from build123d import *

# Parameters (mm, degrees)
SKETCH1_W               = 32
SKETCH1_H               = 80
BOSS_EXTRUDE1_DEPTH     = 3
SKETCH4_W               = 32
SKETCH4_H               = 80
SKETCH4_W_2             = 27
SKETCH4_H_2             = 74
BOSS_EXTRUDE2_DEPTH     = 57.5
SKETCH5_W               = 32
SKETCH5_H               = 140
BOSS_EXTRUDE3_DEPTH     = 2.5
CUT_EXTRUDE1_DEPTH      = 50.8
CUT_EXTRUDE1_DEPTH_BACK = 94.573500522
SKETCH2_W               = 22
SKETCH2_H               = 41
SKETCH6_R               = 3.25
SKETCH6_W               = 22
SKETCH6_H               = 74
CUT_EXTRUDE2_DEPTH      = 25.4
CUT_EXTRUDE3_DEPTH      = 100.463561167
CUT_EXTRUDE3_DEPTH_BACK = 100.463561167
SKETCH8_W               = 74
SKETCH8_H               = 60
SKETCH7_R               = 2
CUT_EXTRUDE4_DEPTH      = 94.573500522
SKETCH10_W              = 2
SKETCH10_H              = 140
CUT_EXTRUDE5_DEPTH      = 96.524865873
FILLET1_R               = 5
SKETCH13_W              = 3
SKETCH13_H              = 41
CUT_EXTRUDE7_DEPTH      = 94.252345815


with BuildPart() as part:
    # Sketch1 → Boss-Extrude1 (new body)
    with BuildSketch(Plane(origin=(0, 0, 0), x_dir=(1, 0, 0), z_dir=(0, 1, 0))):
        with Locations((0, 9)):
            Rectangle(SKETCH1_W, SKETCH1_H)
    extrude(amount=BOSS_EXTRUDE1_DEPTH)

    # Sketch4 → Boss-Extrude2 (add)
    with BuildSketch(Plane(origin=(0, 3, 0), x_dir=(1, 0, 0), z_dir=(0, 1, 0))):
        with Locations((0, 9)):
            Rectangle(SKETCH4_W, SKETCH4_H)
        with Locations((0, 9)):
            Rectangle(SKETCH4_W_2, SKETCH4_H_2, mode=Mode.SUBTRACT)
    extrude(amount=BOSS_EXTRUDE2_DEPTH)

    # Sketch5 → Boss-Extrude3 (add)
    with BuildSketch(Plane(origin=(0, 60.5, 0), x_dir=(1, 0, 0), z_dir=(0, 1, 0))):
        Rectangle(SKETCH5_W, SKETCH5_H)
    extrude(amount=BOSS_EXTRUDE3_DEPTH)

    # Sketch2 → Cut-Extrude1 (cut, two sides: drawn at the far end of the back side and taken through both)
    with BuildSketch(Plane(origin=(0, 3, 0), x_dir=(1, 0, 0), z_dir=(0, 1, 0)).offset(-CUT_EXTRUDE1_DEPTH_BACK)):
        with Locations((0, 9)):
            Rectangle(SKETCH2_W, SKETCH2_H)
    extrude(amount=CUT_EXTRUDE1_DEPTH + CUT_EXTRUDE1_DEPTH_BACK, mode=Mode.SUBTRACT)

    # Sketch6 → Cut-Extrude2 (cut)
    with BuildSketch(Plane(origin=(0, 63, 0), x_dir=(1, 0, 0), z_dir=(0, 1, 0))):
        with Locations(Location((0, 63.5, 0), (0, 0, 270))):
            Circle(SKETCH6_R)
        with Locations(Location((0, -63.5, 0), (0, 0, 270))):
            Circle(SKETCH6_R)
        with Locations((0, 9)):
            Rectangle(SKETCH6_W, SKETCH6_H)
    extrude(amount=-CUT_EXTRUDE2_DEPTH, mode=Mode.SUBTRACT)

    # Sketch8 → Cut-Extrude3 (cut, two sides: drawn at the far end of the back side and taken through both)
    with BuildSketch(Plane(origin=(16, 0, 0), x_dir=(0, 0, -1), z_dir=(1, 0, 0)).offset(-CUT_EXTRUDE3_DEPTH_BACK)):
        with Locations((9, 33)):
            Rectangle(SKETCH8_W, SKETCH8_H)
    extrude(amount=CUT_EXTRUDE3_DEPTH + CUT_EXTRUDE3_DEPTH_BACK, mode=Mode.SUBTRACT)

    # Sketch7 → Cut-Extrude4 (cut, through all)
    with BuildSketch(Plane(origin=(0, 3, 0), x_dir=(1, 0, 0), z_dir=(0, 1, 0))):
        with Locations(Location((-5, 33, 0), (0, 0, 270))):
            Circle(SKETCH7_R)
        with Locations(Location((5, 33, 0), (0, 0, 270))):
            Circle(SKETCH7_R)
        with Locations(Location((-5, -15, 0), (0, 0, 270))):
            Circle(SKETCH7_R)
        with Locations(Location((5, -15, 0), (0, 0, 270))):
            Circle(SKETCH7_R)
    extrude(amount=-CUT_EXTRUDE4_DEPTH, mode=Mode.SUBTRACT)

    # Sketch10 → Cut-Extrude5 (cut, through all)
    with BuildSketch(Plane(origin=(0, 63, 0), x_dir=(1, 0, 0), z_dir=(0, 1, 0))):
        with Locations((-15, 0)):
            Rectangle(SKETCH10_W, SKETCH10_H)
        with Locations((15, 0)):
            Rectangle(SKETCH10_W, SKETCH10_H)
    extrude(amount=-CUT_EXTRUDE5_DEPTH, mode=Mode.SUBTRACT)

    # Fillet1
    fillet1_edges = [part.edges().sort_by_distance(p)[0] for p in [
        (0, 63, -46),
        (0, 60.5, 31),
        (0, 60.5, -49),
        (0, 0, -49),
        (0, 0, 31),
        (0, 3, 28),
        (0, 63, 28),
        (0, 3, -46),
    ]]
    fillet(fillet1_edges, radius=FILLET1_R)

    # Sketch13 → Cut-Extrude7 (cut, through all)
    with BuildSketch(Plane(origin=(0, 3, 0), x_dir=(1, 0, 0), z_dir=(0, 1, 0))):
        with Locations((-12.5, 9)):
            Rectangle(SKETCH13_W, SKETCH13_H)
    extrude(amount=-CUT_EXTRUDE7_DEPTH, mode=Mode.SUBTRACT)


solid = part.part
Here's how the part is built. I have some questions about the finished solid (model axes, mm). A direction names the side the tool comes from. Coordinates: 2 decimals unless noted, no trailing zeros. Write each loop counter-clockwise with the first axis right and the second up, starting at its lowest first coordinate (ties: lowest second). Pieces come first, ordered by that corner, then holes.
Item 1: I want a section at B-B on z = -63.5. Write out the boundary of the cut face in (x, y).
Item 2: If I drill on line 1 (X direction, y = 1.6, z = -33); line 2 (Z direction, x = -6.75, y = 51.5); line 3 (X direction, y = 61.75, z = -63.5), over which ranges is the centre line in solid material (lowest first)?
Item 3: On a 3-axis mill with a long thin cutter (end or side, diameter ignored), from which of +Z, -Z, +X, -X, +Y, -Y can I reach the whole of each face in a straight line? I mean faces 1 (the flat face through (-2, 2, 11.5)), 2 (the flat face through (0, 30, -49)), 3 (the flat face through (12, 3, -9)), 4 (the flat face through (0, 63, 51)), 5 (the cylindrical face through (-5.766, 1.521, -31.153)). Say none if no direction works.
Item 4: If we mould it in two halves opening along Z, with no side actions, what happens to faces 6 (the flat face through (12, 0, -9)), 7 (the cylindrical face through (0, 2, 30)), 8 (the flat face through (0, 33, 28))? For each: +Z half, -Z half, draft (parallel to the pull), parting line (faces both ways), or undercut.
Item 5: I want a section at D-D on y = 47.5. Write out the boundary of the cut face in (x, z), and give its area (3 significant figures).
Item 6: I want a section at C-C on z = -33. Write out the boundary of the cut face in (x, y).
Item 7: I want a section at A-A on x = -5. Count the separate pieces of the cut face and the enclosed holes in it, and give its area (3 significant figures).
Item 8: Will these pins go through, and if not, where does the flat tip stop? pin 1 (8 mm diameter, centred on x = -6, z = -66, fed in from -Y); pin 2 (1.5 mm diameter, centred on x = 7, z = -34, fed in from +Y); pin 3 (4 mm diameter, centred on x = 8.5, y = 52.5, fed in from -Z).
Findings below:
1. outline: (-14, 60.5) - (-3.25, 60.5) - (-3.25, 63) - (-14, 63) - close; (3.25, 60.5) - (14, 60.5) - (14, 63) - (3.25, 63) - close
2. line 1: x = -14 to -7, -3 to 3, 7 to 14
2. line 2: z = -49 to -46, 28 to 31
2. line 3: x = -14 to -3.25, 3.25 to 14
3. face 1: -X, +Y, -Y
3. face 2: -Z, +X, -X, -Y
3. face 3: +X, -X, +Y
3. face 4: +Z, -Z, +X, -X, +Y
3. face 5: +Y, -Y
4. face 6: draft
4. face 7: +Z half
4. face 8: undercut
5. outline: (-14, -49) - (14, -49) - (14, -46) - (-14, -46) - close; (-14, 28) - (14, 28) - (14, 31) - (-14, 31) - close
5. area: 168 mm2
6. outline: (-14, 0) - (-7, 0) - (-7, 3) - (-14, 3) - close; (-3, 0) - (3, 0) - (3, 3) - (-3, 3) - close; (7, 0) - (14, 0) - (14, 3) - (7, 3) - close
7. separate pieces: 4
7. enclosed holes: 0
7. area: 603 mm2
8. pin 1: stops at y = 60.5
8. pin 2: stops at y = 3
8. pin 3: stops at z = -49
